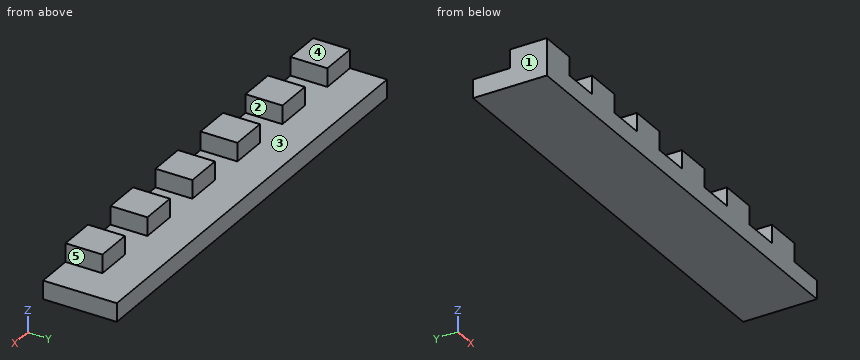
```python
from build123d import *

# Parameters (mm, degrees)
EXTRUDE_1_DEPTH     = 20
SKETCH_2_W          = 5
SKETCH_2_H          = 10
CUT_EXTRUDE_1_DEPTH = 121.099407002


with BuildPart() as part:
    # Эскиз1 → Бобышка-Вытянуть1 (new body)
    with BuildSketch(Plane(origin=(0, 0, 0), x_dir=(1, 0, 0), z_dir=(0, 1, 0))):
        Polygon((0, 0), (10.099407002, 0), (10.099407002, 5), (20.099407002, 5), (20.099407002, 0), (30.099407002, 0), (30.099407002, 5), (40.099407002, 5), (40.099407002, 0), (50.099407002, 0), (50.099407002, 5), (60.099407002, 5), (60.099407002, 0), (70.099407002, 0), (70.099407002, 5), (80.099407002, 5), (80.099407002, 0), (90.099407002, 0), (90.099407002, 5), (100.099407002, 5), (100.099407002, 0), (110.099407002, 0), (110.099407002, 5), (120.099407002, 5), (120.099407002, 10), (0, 10), align=None)
    extrude(amount=EXTRUDE_1_DEPTH)

    # Эскиз2 → Вырез-Вытянуть1 (cut, through all)
    with BuildSketch(Plane.ZY):
        with Locations((-2.5, 15)):
            Rectangle(SKETCH_2_W, SKETCH_2_H)
    extrude(amount=-CUT_EXTRUDE_1_DEPTH, mode=Mode.SUBTRACT)


solid = part.part
```
Model file for the job. Use its own axes, mm. Face numbers are marked on the shaded views. A direction names the side the tool comes from. Coordinates: 2 decimals unless noted, no trailing zeros. Write each loop counter-clockwise with the first axis right and the second up, starting at its lowest first coordinate (ties: lowest second). Pieces come first, ordered by that corner, then holes. Notation, with made-up numbers: (-27.75, 27) - (-13.75, 27) arc R21 cw to (-13.75, 63) - close; hole circle Ø8 at (84, -5). An arc over 180 degrees is marked (long way). One line per item, written item: value. Start each with the question number.
1. Tool access for the marked faces 1 and 2: list every direction of +Z, -Z, +X, -X, +Y, -Y with a clear straight run to the whole face (end or side of a thin tool).
2. Mould opens along X. For the marked faces 3, 4 and 5 say: released by +X, released by -X, zero draft, split by the parting line, or undercut.
3. Slice it at A-A (z = -1.5). Write the cut outline in (x, y), plus the area to 3 significant figures.
4. Flat gauge pins, fed straight in: pin 1 (3 mm diameter, centred on x = 108, z = -1.5, fed in from -Y); pin 2 (4 mm diameter, centred on x = 63, z = -1.5, fed in from +Y); pin 3 (2.5 mm diameter, centred on y = 4.5, z = -3.5, fed in from +X). Where does each tip first touch, or does it go through?
5. Slice it at C-C (x = 27). Write the cut outline in (y, z), plus the area to 3 significant figures.
6. Probe line 1 (X direction, y = 3.25, z = -2.5); line 2 (Y direction, x = 7, z = -4.25); line 3 (Z direction, x = 31, y = 16.5). List the from-to ranges inside material, lowest first. Write a range as from..to.
7. Slice it at B-B (y = 7.5). Write the cut outline in (x, z), plus the area to 3 significant figures.
8. Slice it at D-D (x = 56.5). Write the cut outline in (y, z), plus the area to 3 significant figures.
Answers below:
1. face 1: +Z, -Z, -X, +Y, -Y
1. face 2: +Z, +Y, -Y
2. face 3: undercut
2. face 4: zero draft
2. face 5: released by +X
3. outline: (0, 0) - (10.1, 0) - (10.1, 10) - (0, 10) - close; (20.1, 0) - (30.1, 0) - (30.1, 10) - (20.1, 10) - close; (40.1, 0) - (50.1, 0) - (50.1, 10) - (40.1, 10) - close; (60.1, 0) - (70.1, 0) - (70.1, 10) - (60.1, 10) - close; (80.1, 0) - (90.1, 0) - (90.1, 10) - (80.1, 10) - close; (100.1, 0) - (110.1, 0) - (110.1, 10) - (100.1, 10) - close
3. area: 601 mm^2
4. pin 1: stops at y = 0
4. pin 2: stops at y = 10
4. pin 3: stops at x = 110.1
5. outline: (0, -10) - (20, -10) - (20, -5) - (10, -5) - (10, 0) - (0, 0) - close
5. area: 150 mm^2
6. line 1: x = 0..10.1, 20.1..30.1, 40.1..50.1, 60.1..70.1, 80.1..90.1, 100.1..110.1
6. line 2: y = 0..10
6. line 3: z = -10..-5
7. outline: (0, -10) - (120.1, -10) - (120.1, -5) - (110.1, -5) - (110.1, 0) - (100.1, 0) - (100.1, -5) - (90.1, -5) - (90.1, 0) - (80.1, 0) - (80.1, -5) - (70.1, -5) - (70.1, 0) - (60.1, 0) - (60.1, -5) - (50.1, -5) - (50.1, 0) - (40.1, 0) - (40.1, -5) - (30.1, -5) - (30.1, 0) - (20.1, 0) - (20.1, -5) - (10.1, -5) - (10.1, 0) - (0, 0) - close
7. area: 901 mm^2
8. outline: (0, -10) - (20, -10) - (20, -5) - (0, -5) - close
8. area: 100 mm^2
